The figure shows three views and two pictorial views of one solid part (mm, origin at its lowest corner). Answer the questions. A direction names the side the tool comes from. Coordinates: 2 decimals unless noted, no trailing zeros. Write each loop counter-clockwise with the first axis right and the second up, starting at its lowest first coordinate (ties: lowest second). Pieces come first, ordered by that corner, then holes. Notation, with made-up numbers: M 21,-15.75 L 37,-15.75 A38 ccw 37,23.25 Z; hole C -23.5,44 d5. An arc over 180 degrees is marked long. Write item = value, one per line. Start each with the question number.
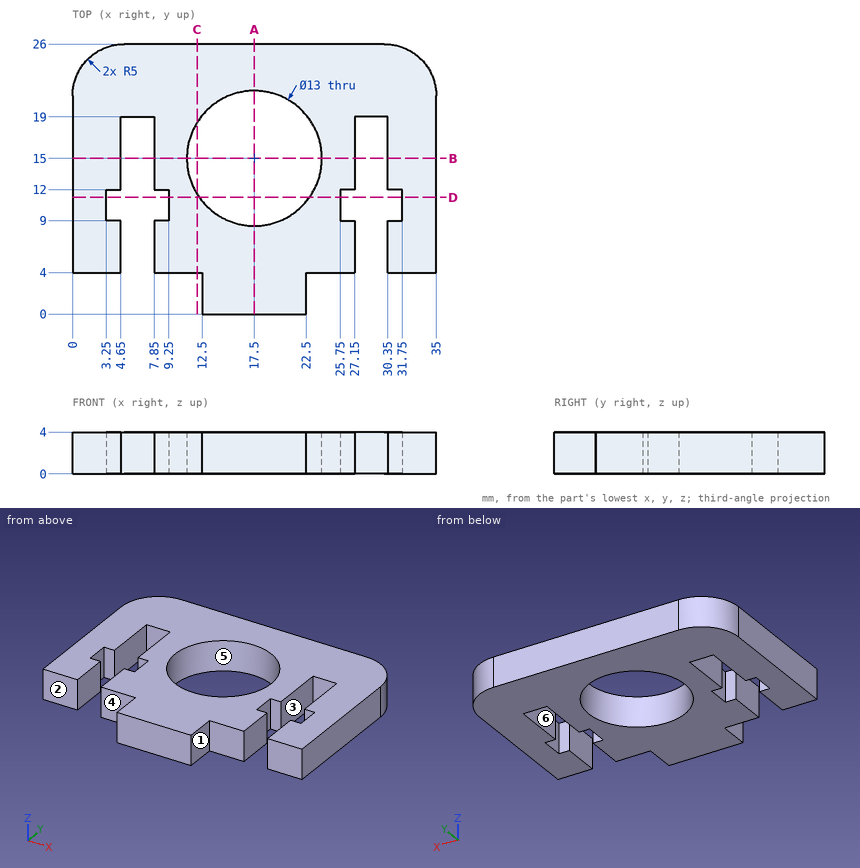
1. For a pull along Y with two mould halves and no side action, classify the marked faces 4, 5 and 6 as pulls with the +Y half, pulls with the -Y half, needs draft (parallel to the pull), parting line crosses it, or undercut.
2. The part is cut by section B-B, the plane y = 15. Write down the section's boundary in (x, z).
3. Each of these flat-tipped pins is pushed along its axis until it touches: pin 1 (2 mm diameter, centred on x = 9, z = 2.5, fed in from -Y); pin 2 (1.6 mm diameter, centred on x = 28.5, z = 2.5, fed in from -Y); pin 3 (1.1 mm diameter, centred on x = 31, z = 2, fed in from +Y). Where does it stop, or does it pass through?
4. The part is cut by section D-D, the plane y = 11.25. Write down the section's boundary in (x, z), and give its area (3 significant figures).
5. Straight lines are drawn through the part: L1, parallel to X at y = 7.5, z = 0.6; L2, parallel to Y at x = 20, z = 3; L3, parallel to X at y = 15.5, z = 1.45. For each, find the intervals that lie inside material, in ascending order. Write a range as [from, to].
6. For the marked faces 1, 2 and 3, determine the directions among +Z, -Z, +X, -X, +Y, -Y from which every point of the face is accessible in a straight line to the end or side of a thin tool.
7. The part is cut by section A-A, the plane x = 17.5. Write down the section's boundary in (y, z), and give its area (3 significant figures).
8. The part is cut by section C-C, the plane x = 12. Write down the section's boundary in (y, z), and give its area (3 significant figures).
Solution:
q1.face_4 = pulls with the -Y half
q1.face_5 = undercut
q1.face_6 = needs draft
q2.outline = M 0,0 L 4.65,0 L 4.65,4 L 0,4 Z; M 7.85,0 L 11,0 L 11,4 L 7.85,4 Z; M 24,0 L 27.15,0 L 27.15,4 L 24,4 Z; M 30.35,0 L 35,0 L 35,4 L 30.35,4 Z
q3.pin_1 = 4
q3.pin_2 = 19
q3.pin_3 = 25.98
q4.outline = M 0,0 L 3.25,0 L 3.25,4 L 0,4 Z; M 9.25,0 L 12.19,0 L 12.19,4 L 9.25,4 Z; M 22.81,0 L 25.75,0 L 25.75,4 L 22.81,4 Z; M 31.75,0 L 35,0 L 35,4 L 31.75,4 Z
q4.area = 49.5 mm^2
q5.L1 = [0, 4.65], [7.85, 27.15], [30.35, 35]
q5.L2 = [0, 9], [21, 26]
q5.L3 = [0, 4.65], [7.85, 11.02], [23.98, 27.15], [30.35, 35]
q6.face_1 = +Z, -Z, +X, -Y
q6.face_2 = +Z, -Z, -X, -Y
q6.face_3 = +Z, -Z, -Y
q7.outline = M 0,0 L 8.5,0 L 8.5,4 L 0,4 Z; M 21.5,0 L 26,0 L 26,4 L 21.5,4 Z
q7.area = 52.0 mm^2
q8.outline = M 4,0 L 11.54,0 L 11.54,4 L 4,4 Z; M 18.46,0 L 26,0 L 26,4 L 18.46,4 Z
q8.area = 60.3 mm^2
